Could you check a few things on this model? Use its own coordinates, in mm. Give positions to 0.01 mm unless a question says otherwise; leave off trailing zeros. Order: outer loops, then holes, each group sorted by start corner. A loop starts at its lowest first (then second) coordinate and runs counter-clockwise, first axis right, second up. Notation, with made-up numbers: M 36,-25.75 L 76,-25.75 A24 cw 76,9.25 Z; hole C 7,69.25 d6. An arc over 180 degrees is marked long. Return JSON: item names as keys, results as strings. Group by question number.
```python
from build123d import *

# Parameters (mm, degrees)
F1_DEPTH = 4
F3_R     = 1.25
F4_DEPTH = 2


with BuildPart() as f1:
    # F0 (on Top) → F1 (new body)
    with BuildSketch(Plane.XY):
        Polygon((21, -30), (25, -30), (35, -30), (35, -22), (25, -22), (25, -14.063702), (36, -14.063702), (36, 19.936298), (0, 19.936298), (0, 15.936298), (32, 15.936298), (32, -10.063702), (0, -10.063702), (0, -14.063702), (21, -14.063702), align=None)
    extrude(amount=F1_DEPTH)

    # F2: F1 across plane


with BuildPart() as f1_1:
    add(f1.part)
    add(f1.part.mirror(Plane.YZ))

    # F3 (on face) → F4 (join)
    with BuildSketch(Plane.XY.offset(4)):
        with BuildLine():
            Line((-32, -3.063702), (-32, -10.063702))
            Line((-32, -10.063702), (-25, -10.063702))
            Line((-25, -10.063702), (-25, -5.563702))
            ThreePointArc((-25, -5.563702), (-25.732233, -3.795935), (-27.5, -3.063702))
            Line((-27.5, -3.063702), (-32, -3.063702))
        make_face()
        with Locations((-28.5, -6.563702)):
            Circle(F3_R, mode=Mode.SUBTRACT)
        with BuildLine():
            Line((-25, 15.936298), (-32, 15.936298))
            Line((-32, 15.936298), (-32, 8.936298))
            Line((-32, 8.936298), (-27.5, 8.936298))
            ThreePointArc((-27.5, 8.936298), (-25.732233, 9.668531), (-25, 11.436298))
            Line((-25, 11.436298), (-25, 15.936298))
        make_face()
        with Locations((-28.5, 12.436298)):
            Circle(F3_R, mode=Mode.SUBTRACT)
        with BuildLine():
            Line((32, 8.936298), (32, 15.936298))
            Line((32, 15.936298), (25, 15.936298))
            Line((25, 15.936298), (25, 11.436298))
            ThreePointArc((25, 11.436298), (25.732233, 9.668531), (27.5, 8.936298))
            Line((27.5, 8.936298), (32, 8.936298))
        make_face()
        with Locations((28.5, 12.436298)):
            Circle(F3_R, mode=Mode.SUBTRACT)
        with BuildLine():
            Line((25, -10.063702), (32, -10.063702))
            Line((32, -10.063702), (32, -3.063702))
            Line((32, -3.063702), (27.5, -3.063702))
            ThreePointArc((27.5, -3.063702), (25.732233, -3.795935), (25, -5.563702))
            Line((25, -5.563702), (25, -10.063702))
        make_face()
        with Locations((28.5, -6.563702)):
            Circle(F3_R, mode=Mode.SUBTRACT)
    extrude(amount=-F4_DEPTH)


solid = f1_1.part
```
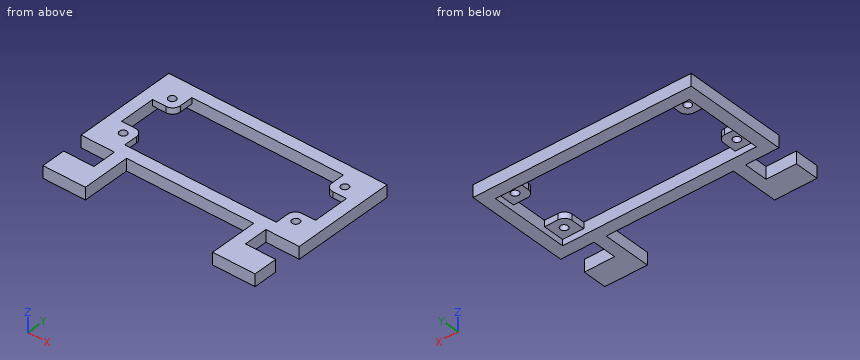
1. Imagine slicing it at C-C, the plane x = -8. Please give me the cut outline in (y, z).
2. I need wall thicknesses on L1, parallel to Y at x = -28.5, z = 2.5; L2, parallel to Y at x = -30.5, z = 1.2; L3, parallel to Y at x = -12, z = 1.4. Which ranges of each line are inside material? Lowest first, please. Write a range as from..to.
3. Imagine slicing it at B-B, the plane y = 15. Please give me the cut outline in (x, z).
4. For pin 1 (2 mm diameter, centred on x = 8, z = 1.5, fed in from -Y); pin 2 (5.5 mm diameter, centred on x = 29, y = 11, fed in from -Z), each with a flat end and sliding along its axis, tell me the tip position at first contact or that it passes through.
5. Imagine slicing it at A-A, the plane x = -28.5. Please give me the cut outline in (y, z).
6. Imagine slicing it at D-D, the plane z = 1.2. Please give me the cut outline in (x, y).
Values:
{
 "1": {"outline": "M -14.06,0 L -10.06,0 L -10.06,4 L -14.06,4 Z; M 15.94,0 L 19.94,0 L 19.94,4 L 15.94,4 Z"},
 "2": {"L1": "y = -30..-22, -14.06..-7.81, -5.31..-3.06, 8.94..11.19, 13.69..19.94", "L2": "y = -30..-22, -14.06..-10.06, 15.94..19.94", "L3": "y = -14.06..-10.06, 15.94..19.94"},
 "3": {"outline": "M -36,0 L -32,0 L -32,2 L -25,2 L -25,4 L -36,4 Z; M 25,2 L 32,2 L 32,0 L 36,0 L 36,4 L 25,4 Z"},
 "4": {"pin 1": "stops at y = -14.06", "pin 2": "stops at z = 2"},
 "5": {"outline": "M -30,0 L -22,0 L -22,4 L -30,4 Z; M -14.06,0 L -10.06,0 L -10.06,2 L -7.81,2 L -7.81,4 L -14.06,4 Z; M -5.31,2 L -3.06,2 L -3.06,4 L -5.31,4 Z; M 8.94,2 L 11.19,2 L 11.19,4 L 8.94,4 Z; M 13.69,2 L 15.94,2 L 15.94,0 L 19.94,0 L 19.94,4 L 13.69,4 Z"},
 "6": {"outline": "M -36,-14.06 L -25,-14.06 L -25,-22 L -35,-22 L -35,-30 L -21,-30 L -21,-14.06 L 21,-14.06 L 21,-30 L 35,-30 L 35,-22 L 25,-22 L 25,-14.06 L 36,-14.06 L 36,19.94 L -36,19.94 Z; hole M -32,-10.06 L 32,-10.06 L 32,15.94 L -32,15.94 Z"}
}
